from build123d import *

# Parameters (mm, degrees)
F0_R      = 59.457359
F1_DEPTH  = 12.7
F3_R      = 26.633643
F4_DEPTH  = 12.7
F5_W      = 408.406466
F5_H      = 13.974104
F6_DEPTH  = 177.8
F7_R      = 25.770774
F8_DEPTH  = 12.7
F9_R      = 57.38091
F10_DEPTH = 12.7
F11_W     = 27.406466
F11_H     = 88.9
F12_DEPTH = 6.35
F13_R     = 23.109581
F14_DEPTH = 12.7
F15_R     = 63.126409
F16_DEPTH = 12.7
F17_R     = 23.353727
F18_DEPTH = 12.7
F19_R     = 63.420854
F20_DEPTH = 12.7
F22_DEPTH = 31.75
F24_D     = 12.7
F26_D     = 12.7


with BuildPart() as f1:
    # F0 (on Front) → F1 (new body)
    with BuildSketch(Plane.XZ):
        with Locations((-52.107409, 44.159733)):
            Circle(F0_R)
    extrude(amount=F1_DEPTH)

    # F3 (on face) → F4 (join)
    with BuildSketch(Plane.XZ.offset(12.7)):
        with Locations((-60.155295, 49.909814)):
            Circle(F3_R)
    extrude(amount=F4_DEPTH)

    # F5 (on face) → F6 (join)
    with BuildSketch(Plane.XZ.offset(25.4)):
        with Locations((62.345162, 47.209637)):
            Rectangle(F5_W, F5_H)
    extrude(amount=F6_DEPTH)

    # F7 (on face) → F8 (join)
    with BuildSketch(Plane.XZ.offset(203.2)):
        with Locations((-55.428505, 44.736113)):
            Circle(F7_R)
    extrude(amount=F8_DEPTH)

    # F9 (on face) → F10 (join)
    with BuildSketch(Plane.XZ.offset(215.9)):
        with Locations((-55.428505, 44.736113)):
            Circle(F9_R)
    extrude(amount=F10_DEPTH)

    # F11 (on face) → F12 (join)
    with BuildSketch(Plane.XY.offset(54.196689)):
        with Locations((-77.354838, -107.95)):
            Rectangle(F11_W, F11_H)
    extrude(amount=F12_DEPTH)

    # F13 (on face) → F14 (join)
    with BuildSketch(Plane.XZ.offset(203.2)):
        with Locations((214.701638, 47.041636)):
            Circle(F13_R)
    extrude(amount=F14_DEPTH)

    # F15 (on face) → F16 (join)
    with BuildSketch(Plane.XZ.offset(215.9)):
        with Locations((214.701638, 47.041636)):
            Circle(F15_R)
    extrude(amount=F16_DEPTH)

    # F17 (on face) → F18 (join)
    with BuildSketch(Plane(origin=(0, -25.4, 0), x_dir=(-1, 0, 0), z_dir=(0, 1, 0))):
        with Locations((-214.270413, 47.866244)):
            Circle(F17_R)
    extrude(amount=F18_DEPTH)

    # F19 (on face) → F20 (join)
    with BuildSketch(Plane(origin=(0, -12.7, 0), x_dir=(-1, 0, 0), z_dir=(0, 1, 0))):
        with Locations((-214.270413, 47.866244)):
            Circle(F19_R)
    extrude(amount=F20_DEPTH)

    # F21 (on face) → F22 (join)
    with BuildSketch(Plane.XY.offset(54.196689)):
        Polygon((143.312216, -42.225428), (-22.581015, -42.225428), (-23.332113, -55.224109), (125.416026, -55.224109), (125.416026, -176.853418), (-25.890864, -176.853418), (-25.890864, -193.850324), (143.312216, -193.850324), align=None)
    extrude(amount=F22_DEPTH)

    # F24 (through all)
    with Locations(Plane.XZ.offset(228.6)):
        with Locations((-55.428505, 44.736113)):
            Hole(F24_D / 2)

    # F26 (through all)
    with Locations(Plane.XZ.offset(228.6)):
        with Locations((214.701638, 47.041636)):
            Hole(F26_D / 2)


solid = f1.part
The listing builds one solid part. Answer for the finished solid, in the listing's coordinates (mm). A direction names the side the tool comes from. Coordinates: 2 decimals unless noted, no trailing zeros. Write each loop counter-clockwise with the first axis right and the second up, starting at its lowest first coordinate (ties: lowest second). Pieces come first, ordered by that corner, then holes. Notation, with made-up numbers: (29.5, 35.5) - (63.5, 35.5) arc R11 cw to (63.5, 50.5) - close; hole circle Ø10 at (-15.75, 60.25). An arc over 180 degrees is marked (long way). Put each result on its own line as item: value.
1. The part is cut by section D-D on x = 72.5. Give the vertices of the cut face in (y, z).
Answer sheet:
outline: (-203.2, 40.22) - (-25.4, 40.22) - (-25.4, 54.2) - (-42.23, 54.2) - (-42.23, 85.95) - (-55.22, 85.95) - (-55.22, 54.2) - (-176.85, 54.2) - (-176.85, 85.95) - (-193.85, 85.95) - (-193.85, 54.2) - (-203.2, 54.2) - close
2. A tool of negligible diameter and unlimited length cuts with its end or side. For faces 1 (the face through (77, -25.4, 47)), 2 (the face through (-111.507, -6.261, 46.774)), 3 (the face through (-101, -113, 40.223)), 4 (the face through (51, -176.853, 70)), from which of +Z, -Z, +X, -X, +Y, -Y can it reach the whole face along a straight path? Write none if from no direction.
Answer sheet:
face 1: +Z, -Z
face 2: +Y
face 3: -Z, +X, -X
face 4: +Z, -X
3. Find the intervals of material crossed by line 1 along Y through (x, z) = (-58.5, 5); line 2 along X through (y, z) = (-214, 49); line 3 along Z through (x, y) = (72, -85.5), in increasing order. Write a range as from..to.
Answer sheet:
line 1: y = -228.6..-215.9, -12.7..0
line 2: x = -80.84..-60.13, -50.72..-30.01, 191.68..208.66, 220.74..237.73
line 3: z = 40.22..54.2
4. Determine the mould class of faces 5 (the face through (-2.423, -222.161, 22.759)), 6 (the face through (79, -203.2, 47)), 7 (the face through (215, 0, 35)) for opening direction Y: pulls with the +Y half, pulls with the -Y half, needs draft (parallel to the pull), parting line crosses it, or undercut.
Answer sheet:
face 5: needs draft
face 6: undercut
face 7: pulls with the +Y half
5. The part is cut by section A-A on z = 8.5. Give the vertices of the cut face in (x, y).
Answer sheet:
outline: (-99.92, -228.6) - (-10.94, -228.6) - (-10.94, -215.9) - (-99.92, -215.9) - close; (-99.68, -12.7) - (-4.53, -12.7) - (-4.53, 0) - (-99.68, 0) - close; (164.55, -12.7) - (263.99, -12.7) - (263.99, 0) - (164.55, 0) - close; (164.71, -228.6) - (264.7, -228.6) - (264.7, -215.9) - (164.71, -215.9) - close
6. The part is cut by section B-B on x = 184.5. Give the vertices of the cut face in (y, z), plus the area to 3 significant figures.
Answer sheet:
outline: (-228.6, -8.39) - (-215.9, -8.39) - (-215.9, 102.47) - (-228.6, 102.47) - close; (-203.2, 40.22) - (-25.4, 40.22) - (-25.4, 54.2) - (-203.2, 54.2) - close; (-12.7, -8.13) - (0, -8.13) - (0, 103.87) - (-12.7, 103.87) - close
area: 5,310 mm^2
7. Flat-ended cylindrical pins translate along their axes: pin 1 Ø10 at (x, z) = (133.5, 88.5) entering from +Y; pin 2 Ø2 at (x, y) = (-62.5, -115) entering from +Z; pin 3 Ø6 at (y, z) = (-79, 81.5) entering from -X; pin 4 Ø2 at (y, z) = (-157, 88.5) entering from -X. Find the tip coordinate at first contact, or state that the pin passes through.
Answer sheet:
pin 1: stops at y = -42.23
pin 2: stops at z = 54.2
pin 3: stops at x = 125.42
pin 4: passes through
8. The part is cut by section C-C on y = -135.5. Give the vertices of the cut face in (x, z).
Answer sheet:
outline: (-141.86, 40.22) - (-59.9, 40.22) arc R6.35 cw (long way) to (-50.96, 40.22) - (266.55, 40.22) - (266.55, 54.2) - (143.31, 54.2) - (143.31, 85.95) - (125.42, 85.95) - (125.42, 54.2) - (-63.65, 54.2) - (-63.65, 60.55) - (-91.06, 60.55) - (-91.06, 54.2) - (-141.86, 54.2) - close; hole circle Ø12.7 at (214.7, 47.04)
